Autodesk Fusion 360 part; units mm, degrees
sketch "Sketch1" plane through (0, 0, 0) normal (0, 0, 1) x (1, 0, 0)
  line L0 (-50, 25) -> (28, 25)
  line L1 (28, 25) -> (28, -31)
  line L2 (28, -31) -> (-50, -31)
  line L3 (-50, -31) -> (-50, 25)
  line L4 (-55, 30) -> (30, 30)
  line L5 (30, 30) -> (30, -35)
  line L6 (30, -35) -> (-55, -35)
  line L7 (-55, -35) -> (-55, 30)
  dimension "d1" = 78
  dimension "d2" = 56
extrude "Extrude1" add sketch "Sketch1" along normal blind 3
sketch "Sketch2" plane through (0, 0, 3) normal (0, 0, 1) x (-1, 0, 0)
  line L0 (-28, 31) -> (50, 31)
  line L1 (50, 31) -> (50, -25)
  line L2 (50, -25) -> (-28, -25)
  line L3 (-28, -25) -> (-28, 31)
  line L4 (55, 35) -> (-30, 35)
  line L5 (-30, 35) -> (-30, -30)
  line L6 (-30, -30) -> (55, -30)
  line L7 (55, -30) -> (55, 35)
  line L8 (50, -25) -> (-28, -25)
  line L9 (-28, -25) -> (-28, -30)
  line L10 (-28, -30) -> (50, -30)
  line L11 (50, -30) -> (50, -25)
  line L12 (-28, 31) -> (50, 31)
  line L13 (50, 31) -> (50, 35)
  line L14 (50, 35) -> (-28, 35)
  line L15 (-28, 35) -> (-28, 31)
extrude "Extrude2" add sketch "Sketch2" along normal blind 5 contours L0 L4 L12 L13 L14 L15 | L2 L6 L8 L9 L10 L11
extrude "Extrude3" add 1 faces at (30, 8.3333, 1) along direction (1, 0, 0) blind 4
extrude "Extrude4" add 1 faces at (-55, -13.3333, 1) along direction (-1, 0, 0) blind 1
sketch "Sketch3" plane through (0, 0, 3) normal (0, 0, 1) x (-1, 0, 0)
  line L0 (50, 35) -> (50, 31)
  line L1 (50, 31) -> (50, -25)
  line L2 (50, -25) -> (50, -30)
  line L3 (50, -30) -> (56, -30)
  line L4 (56, -30) -> (56, 35)
  line L5 (56, 35) -> (50, 35)
  circle A0 centre (53, -21.75) radius 1.25
  circle A1 centre (-31, -21.75) radius 1.25
  circle A2 centre (-31, 27.75) radius 1.25
  circle A3 centre (53, 27.75) radius 1.25
  dimension "d11" = 2.5
  dimension "d12" = 2.5
  dimension "d13" = 2.5
  dimension "d14" = 2.5
extrude "Extrude5" add sketch "Sketch3" along normal blind 3 contours A0 | A1 | A2 | A3
extrude "Extrude6" add 2 faces at (2, 28.3333, 8) (2, -32.3333, 8) along direction (0, 0, 1) blind 1
extrude "Extrude7" cut 1 faces at (-24, 30, 7) along direction (0, -1, 0) blind 2
extrude "Extrude8" cut 1 faces at (-24, -35, 5) along direction (0, 1, 0) blind 1
sketch "Sketch4" plane through (0, 0, 3) normal (0, 0, 1) x (-1, 0, 0)
  line L0 (56, 34) -> (50, 34)
  line L1 (50, 34) -> (50, 31)
  line L2 (50, 31) -> (50, -25)
  line L3 (50, -25) -> (50, -28)
  line L4 (50, -28) -> (56, -28)
  line L5 (56, -28) -> (56, 34)
  circle A0 centre (53, -21.75) radius 1.25
  circle A1 centre (53, 27.75) radius 1.25
  line L6 (50, -17) -> (54, -17)
  line L7 (54, -17) -> (54, 23)
  line L8 (54, 23) -> (50, 23)
  line L9 (50, 23) -> (50, -17)
extrude "Extrude9" cut sketch "Sketch4" against normal blind 2.5 contours L2 L6 L7 L8 L9
extrude "Extrude10" add 2 faces at (-50, -32, 5) (-50, 26, 5) along direction (-1, 0, 0) up to surface end surface through (-56, -35, 0) normal (-1, 0, 0) offset 0
extrude "Extrude11" add 2 faces at (28, -32, 7) (28, 26, 5) along direction (1, 0, 0) up to surface end surface through (34, 30, 0) normal (1, 0, 0) offset 0
extrude "Extrude12" cut 2 faces at (4, 26, 9) (4, -33, 9) along direction (0, 0, -1) blind 0.5
chamfer "Chamfer1" distance 5 angle 45 1 edges at (-56, 26.5, 8.5)
fillet "Fillet4" radius 3 3 edges at (-56, -34, 4.25) (34, -34, 4.25) (34, 28, 4.25)
sketch "Sketch5" plane through (0, -34, 0) normal (0, -1, 0) x (1, 0, 0)
  line L0 (31, 0) -> (31, 8.5)
  line L1 (31, 8.5) -> (-53, 8.5)
  line L2 (-53, 8.5) -> (-53, 0)
  line L3 (-53, 0) -> (31, 0)
  line L4 (-56, 0) -> (-34, 0)
  line L5 (-34, 0) -> (-34, 10.214)
  line L6 (-34, 10.214) -> (-12, 10.214)
  line L7 (-12, 10.214) -> (-12, -0.4704)
  line L8 (-12, -0.4704) -> (-34, -0.4704)
  line L9 (-34, -0.4704) -> (-34, 0)
  point P0 (-56, 0)
  dimension "d40" = 90
  dimension "d41" = 22
extrude "Extrude13" cut sketch "Sketch5" against normal blind 2 contours L1 L3 L5 L7
fillet "Fillet5" radius 1 2 edges at (-34, -34, 4.25) (-12, -34, 4.25)
extrude "Extrude14" add 1 faces at (-54, 7.3331, 0) along direction (0, 0, -1) blind 0.25
Check sheet for the modelled part. Datum: model origin and axes. Units: mm. A direction names the side the tool comes from. Give positions to 0.01 mm unless a question says otherwise; leave off trailing zeros. Write each loop counter-clockwise with the first axis right and the second up, starting at its lowest first coordinate (ties: lowest second). Pieces come first, ordered by that corner, then holes. Notation, with made-up numbers: (48, 57) - (57, 57) arc R20 ccw to (57, 82) - close; hole circle Ø8 at (25, 45.25). An arc over 180 degrees is marked (long way). Answer as a JSON object with one key per item and string values. Group by question number.
1) Access from +Z, -Z, +X, -X, +Y, -Y to the whole of each face (thin tool, end or side, straight path). Record for faces 4 (the face through (31, 22, 6)), 5 (the face through (-50, -3, 0)), 6 (the face through (-54, -27, 4)).
2) Sectioned sample at C-C (z = 1.75). Record the cut outline in (x, y).
3) Sectioned sample at D-D (y = -27.75). Record the cut outline in (x, z).
4) Depth check by flat-ended pin: P1, Ø6.5, axis at x = -52, y = 11, coming from the +Z side; P2, Ø0.5, axis at y = -32.5, z = 5.5, coming from the +X side; P3, Ø2, axis at y = -22.5, z = 4.5, coming from the -X side; P4, Ø3, axis at x = -51.5, y = -6, coming from the +Z side. Enter the tip coordinate at first touch or a pass-through.
5) Sectioned sample at B-B (y = -9). Record the cut outline in (x, z), then the cut area to 3 significant figures.
6) Sectioned sample at A-A (x = 24). Record the cut outline in (y, z), then the cut area to 3 significant figures.
7) Release check for a two-part mould opening along Y. For faces 1 (the face through (10, -34, 4)), 2 (the face through (34, -3, 2)), 3 (the face through (-54.3, -3.4, 3)) record: pulls with the +Y half, pulls with the -Y half, needs draft (parallel to the pull), parting line crosses it, or undercut.
8) Thickness scan on probe 1 along Y at (x, z) = (-8, 5.25); probe 2 along X at (y, z) = (24.5, 2.5); probe 3 along Y at (x, z) = (-30, 6.5). Record the ranges inside material, lowest first. Write a range as from..to.
Geometry results:
{
 "1": {"face 4": "+Z, +X, -X", "face 5": "+Z, -Z", "face 6": "+Z"},
 "2": {"outline": "(-56, -31) arc R3 ccw to (-53, -34) - (-35, -34) arc R1 ccw to (-34, -33) - (-34, -32) - (-12, -32) - (-12, -33) arc R1 ccw to (-11, -34) - (31, -34) arc R3 ccw to (34, -31) - (34, 25) arc R3 ccw to (31, 28) - (-56, 28) - close; hole (-54, -23) - (-50, -23) - (-50, -31) - (28, -31) - (28, 25) - (-50, 25) - (-50, 17) - (-54, 17) - close"},
 "3": {"outline": "(-56, -0.25) - (-50, -0.25) - (-50, 3) - (-51.75, 3) - (-51.75, 6) - (-54.25, 6) - (-54.25, 3) - (-56, 3) - close; (28, -0.25) - (34, -0.25) - (34, 3) - (32.25, 3) - (32.25, 6) - (29.75, 6) - (29.75, 3) - (28, 3) - close"},
 "4": {"P1": "stops at z = 3", "P2": "stops at x = 33.73", "P3": "passes through", "P4": "stops at z = 0.5"},
 "5": {"outline": "(-56, -0.25) - (-50, -0.25) - (-50, 0.5) - (-54, 0.5) - (-54, 3) - (-56, 3) - close; (28, -0.25) - (34, -0.25) - (34, 3) - (28, 3) - close", "area": "29.0 mm^2"},
 "6": {"outline": "(-34, -0.25) - (-31, -0.25) - (-31, 8.5) - (-34, 8.5) - close; (25, -0.25) - (28, -0.25) - (28, 8.5) - (25, 8.5) - close", "area": "52.5 mm^2"},
 "7": {"face 1": "pulls with the -Y half", "face 2": "needs draft", "face 3": "undercut"},
 "8": {"probe 1": "y = -34..-31, 25..28", "probe 2": "x = -56..-50, 28..34", "probe 3": "y = -32..-31, 25..28"}
}
